Model file for the job. Use its own axes, mm. Give positions to 0.01 mm unless a question says otherwise; leave off trailing zeros. Write each loop counter-clockwise with the first axis right and the second up, starting at its lowest first coordinate (ties: lowest second). Pieces come first, ordered by that corner, then holes. Notation, with made-up numbers: (63.5, 53) - (113.5, 53) arc R28 cw to (113.5, 75) - close; hole circle Ø6 at (-10, 46.25). An arc over 180 degrees is marked (long way). One line per item, written item: value. Start each with the question number.
(1) Cut at D-D, the plane y = 152. List the corners of the cut face in (x, z).
(2) Cut at C-C, the plane x = 3. List the corners of the cut face in (y, z).
(3) Cut at A-A, the plane y = 189.5. List the corners of the cut face in (x, z), and give its area (3 significant figures).
(4) Cut at B-B, the plane z = -40.77. List the corners of the cut face in (x, y), and give its area (3 significant figures).
(5) Probe L1, parallel to Y at x = 7, z = -25; L2, parallel to Y at x = 7.25, z = -40.77; L3, parallel to Z at x = 3.5, y = 173.73. List the from-to ranges inside material, lowest first.
(6) Drop flat-ended pins along their axis: P1, Ø5, axis at x = 7, z = -71, coming from the +Y side; P2, Ø3, axis at x = 4, y = 124, coming from the +Z side; P3, Ø4.5, axis at y = 152, z = -25, coming from the -X side; P4, Ø1.5, axis at x = 5.5, y = 201, coming from the -Z side. Give the stop position or say it passes through.
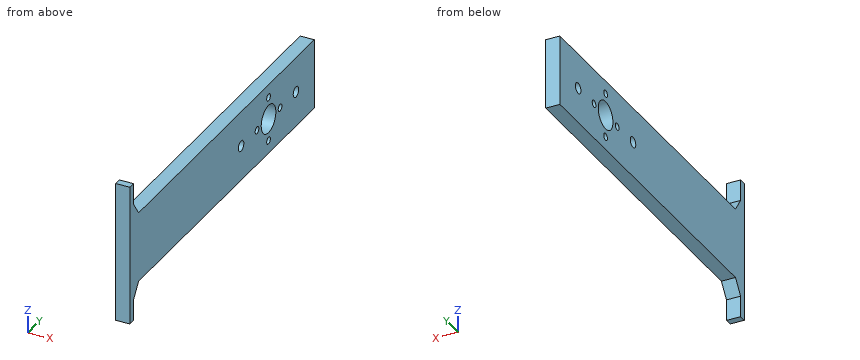
from build123d import *

# Parameters (mm, degrees)
BOSS_EXTRUDE1_DEPTH = 252
CUT_EXTRUDE2_DEPTH  = 10
SKETCH4_W           = 25
SKETCH4_H           = 52
CUT_EXTRUDE3_DEPTH  = 10
SKETCH5_R           = 3.75
SKETCH5_R_2         = 10
CUT_EXTRUDE5_DEPTH  = 264.114043715
SKETCH6_R           = 2.5
CUT_EXTRUDE6_DEPTH  = 264.114043715


with BuildPart() as part:
    # Sketch1 → Boss-Extrude1 (new body)
    with BuildSketch(Plane(origin=(0, 0, 0), x_dir=(1, 0, 0), z_dir=(0, 1, 0))):
        Polygon((10, 0), (10, 50), (10, 75), (0, 75), (0, 50), (0, 0), (0, -25), (10, -25), align=None)
    extrude(amount=BOSS_EXTRUDE1_DEPTH)

    # Sketch3 → Cut-Extrude2 (cut)
    with BuildSketch(Plane.ZY):
        Polygon((25, 200), (25, 5), (10, 5), (0, 11.937821542), (0, 200), align=None)
        Polygon((-75, 5), (-60, 5), (-50, 11.937821542), (-50, 252), (-75, 252), align=None)
    extrude(amount=-CUT_EXTRUDE2_DEPTH, mode=Mode.SUBTRACT)

    # Sketch4 → Cut-Extrude3 (cut)
    with BuildSketch(Plane(origin=(10, 0, 0), x_dir=(0, 0, -1), z_dir=(1, 0, 0))):
        with Locations((-12.5, 226)):
            Rectangle(SKETCH4_W, SKETCH4_H)
    extrude(amount=-CUT_EXTRUDE3_DEPTH, mode=Mode.SUBTRACT)

    # Sketch5 → Cut-Extrude5 (cut, through all)
    with BuildSketch(Plane(origin=(10, 0, 0), x_dir=(0, 0, -1), z_dir=(1, 0, 0))):
        with Locations((25, 227)):
            Circle(SKETCH5_R)
        with Locations((25, 189.5)):
            Circle(SKETCH5_R_2)
        with Locations(Location((25, 152, 0), (0, 0, 180))):
            Circle(SKETCH5_R)
    extrude(amount=-CUT_EXTRUDE5_DEPTH, mode=Mode.SUBTRACT)

    # Sketch6 → Cut-Extrude6 (cut, through all)
    with BuildSketch(Plane.ZY):
        with Locations((-40.77, 189.5)):
            Circle(SKETCH6_R)
        with Locations(Location((-9.23, 189.5, 0), (0, 0, 180))):
            Circle(SKETCH6_R)
        with Locations((-25, 205.27)):
            Circle(SKETCH6_R)
        with Locations(Location((-25, 173.73, 0), (0, 0, 180))):
            Circle(SKETCH6_R)
    extrude(amount=-CUT_EXTRUDE6_DEPTH, mode=Mode.SUBTRACT)


solid = part.part
Answers follow:
1. outline: (0, -50) - (10, -50) - (10, -28.75) - (0, -28.75) - close; (0, -21.25) - (10, -21.25) - (10, 0) - (0, 0) - close
2. outline: (0, -75) - (5, -75) - (5, -60) - (11.94, -50) - (252, -50) - (252, 0) - (11.94, 0) - (5, 10) - (5, 25) - (0, 25) - close; hole circle Ø7.5 at (152, -25); hole circle Ø5 at (173.73, -25); hole circle Ø20 at (189.5, -25); hole circle Ø5 at (189.5, -40.77); hole circle Ø5 at (189.5, -9.23); hole circle Ø5 at (205.27, -25); hole circle Ø7.5 at (227, -25)
3. outline: (0, -50) - (10, -50) - (10, -43.27) - (0, -43.27) - close; (0, -38.27) - (10, -38.27) - (10, -35) - (0, -35) - close; (0, -15) - (10, -15) - (10, -11.73) - (0, -11.73) - close; (0, -6.73) - (10, -6.73) - (10, 0) - (0, 0) - close
3. area: 200 mm²
4. outline: (0, 0) - (10, 0) - (10, 187) - (0, 187) - close; (0, 192) - (10, 192) - (10, 252) - (0, 252) - close
4. area: 2,470 mm²
5. L1: y = 0 to 148.25, 155.75 to 171.23, 176.23 to 179.5, 199.5 to 202.77, 207.77 to 223.25, 230.75 to 252
5. L2: y = 0 to 187, 192 to 252
5. L3: z = -50 to -27.5, -22.5 to 0
6. P1: stops at y = 5
6. P2: stops at z = 0
6. P3: passes through
6. P4: stops at z = -50
